Model file for the job. Use its own axes, mm. A direction names the side the tool comes from. Round coordinates to 2 decimals unless told otherwise and drop trailing zeros. Loops run counter-clockwise (first coordinate to the right, second up) from the corner with the lowest first, then second, coordinate; pieces in that order, holes last. Notation, with made-up numbers: (68, 26) - (112, 26) arc R11 ccw to (112, 31) - close; hole circle Ø7 at (65, 38). An arc over 180 degrees is marked (long way). Answer as a JSON object with one key per item and string values.
from build123d import *

# Parameters (mm, degrees)
EXTRUDE_1_DEPTH             = 25
SKETCH_2_W                  = 1
SKETCH_2_H                  = 50
CUT_EXTRUDE_1_DEPTH         = 26
SKETCH_3_W                  = 52
SKETCH_3_H                  = 1
EXTRUDE_2_DEPTH             = 25
SKETCH_4_W                  = 2
SKETCH_4_H                  = 1
EXTRUDE_3_DEPTH             = 25
SKETCH_5_W                  = 2
SKETCH_5_H                  = 1
EXTRUDE_4_DEPTH             = 25
SKETCH_6_W                  = 11
SKETCH_6_H                  = 1
CUT_EXTRUDE_2_DEPTH         = 26
SKETCH_7_R                  = 8.5
CUT_EXTRUDE_3_DEPTH         = 64
SKETCH_8_R                  = 9.5
CUT_EXTRUDE_4_DEPTH         = 5
SKETCH_9_W                  = 2
SKETCH_9_H                  = 5
EXTRUDE_5_DEPTH             = 25
HOLE_WIZARD_1_D             = 3.4
HOLE_WIZARD_1_DEPTH         = 5
HOLE_WIZARD_1_CBORE_D       = 6
HOLE_WIZARD_1_CBORE_DEPTH   = 3
SKETCH_14_R                 = 1.5
CUT_EXTRUDE_8_DEPTH         = 5
SKETCH_22_W                 = 25
SKETCH_22_H                 = 52
EXTRUDE_9_DEPTH             = 2
CUT_EXTRUDE_START           = -6
CUT_EXTRUDE_10_DEPTH        = 6
CUT_EXTRUDE_11_REACH        = 173
SKETCH_17_R                 = 7.5
CUT_EXTRUDE_12_DEPTH        = 60
HOLE_WIZARD_M3_1_D          = 2.5
HOLE_WIZARD_M3_1_DEPTH      = 8.5
HOLE_WIZARD_M3_1_TIP        = 0.751075774
HOLE_WIZARD_M3_2_AT_2_COUNT = 2
HOLE_WIZARD_M3_2_AT_2_PITCH = 8.5
HOLE_WIZARD_M3_2_AT_3_COUNT = 2
HOLE_WIZARD_M3_2_AT_3_PITCH = 17


with BuildPart() as part:
    # 草图1 → 凸台-拉伸1 (new body)
    with BuildSketch(Plane.XY):
        Polygon((-81, -29), (86, -29), (86, -34), (-86, -34), (-86, -29), (-86, 29), (-81, 29), align=None)
    extrude(amount=EXTRUDE_1_DEPTH)

    # 草图2 → 切除-拉伸1 (cut, through all)
    with BuildSketch(Plane.XY.offset(25)):
        with Locations((-85.5, 0)):
            Rectangle(SKETCH_2_W, SKETCH_2_H)
    extrude(amount=-CUT_EXTRUDE_1_DEPTH, mode=Mode.SUBTRACT)

    # 草图3 → 凸台-拉伸2 (add)
    with BuildSketch(Plane.XY.offset(25)):
        with Locations((0, -28.5)):
            Rectangle(SKETCH_3_W, SKETCH_3_H)
    extrude(amount=-EXTRUDE_2_DEPTH)

    # 草图4 → 凸台-拉伸3 (add)
    with BuildSketch(Plane.XY.offset(25)):
        with Locations((-80, -28.5)):
            Rectangle(SKETCH_4_W, SKETCH_4_H)
    extrude(amount=-EXTRUDE_3_DEPTH)

    # 草图5 → 凸台-拉伸4 (add)
    with BuildSketch(Plane.XY.offset(25)):
        with Locations((78, -28.5)):
            Rectangle(SKETCH_5_W, SKETCH_5_H)
    extrude(amount=-EXTRUDE_4_DEPTH)

    # 草图6 → 切除-拉伸2 (cut, through all)
    with BuildSketch(Plane.XY.offset(25)):
        with Locations((-20.5, -33.5)):
            Rectangle(SKETCH_6_W, SKETCH_6_H)
    cut_extrude_2 = extrude(amount=-CUT_EXTRUDE_2_DEPTH, mode=Mode.SUBTRACT)

    # 镜向1: 切除-拉伸2 across plane
    add(cut_extrude_2.mirror(Plane(origin=(0, 0, 0), x_dir=(0, 0, 1), z_dir=(1, 0, 0))), mode=Mode.SUBTRACT)

    # 草图7 → 切除-拉伸3 (cut, through all)
    with BuildSketch(Plane.XZ.offset(34)):
        with Locations((0, 12.5)):
            Circle(SKETCH_7_R)
    extrude(amount=-CUT_EXTRUDE_3_DEPTH, mode=Mode.SUBTRACT)

    # 草图8 → 切除-拉伸4 (cut)
    with BuildSketch(Plane(origin=(0, -28, 0), x_dir=(1, 0, 0), z_dir=(0, 1, 0))):
        with Locations((0, -12.5)):
            Circle(SKETCH_8_R)
    extrude(amount=-CUT_EXTRUDE_4_DEPTH, mode=Mode.SUBTRACT)

    # 草图9 → 凸台-拉伸5 (add)
    with BuildSketch(Plane(origin=(0, 0, 0), x_dir=(-1, 0, 0), z_dir=(0, 0, -1))):
        with Locations((80, 26.5)):
            Rectangle(SKETCH_9_W, SKETCH_9_H)
    extrude(amount=-EXTRUDE_5_DEPTH)

    # 孔1
    with Locations(Plane(origin=(82.5, -34, 21), x_dir=(-1, 0, 0), z_dir=(0, -1, 0))):
        with Locations((0, 0), (0, 8.5), (0, 17)):
            CounterBoreHole(HOLE_WIZARD_1_D / 2, HOLE_WIZARD_1_CBORE_D / 2, HOLE_WIZARD_1_CBORE_DEPTH, depth=HOLE_WIZARD_1_DEPTH)

    # 草图14 → 切除-拉伸8 (cut)
    with BuildSketch(Plane.XZ.offset(33)):
        with Locations((-23, 20)):
            Circle(SKETCH_14_R)
        with Locations((-23, 5)):
            Circle(SKETCH_14_R)
    cut_extrude_8 = extrude(amount=-CUT_EXTRUDE_8_DEPTH, mode=Mode.SUBTRACT)

    # 镜向2: 切除-拉伸8 across plane
    add(cut_extrude_8.mirror(Plane(origin=(0, 0, 0), x_dir=(0, 0, 1), z_dir=(1, 0, 0))), mode=Mode.SUBTRACT)

    # 草图22 → 凸台-拉伸9 (add)
    with BuildSketch(Plane(origin=(-81, 0, 0), x_dir=(0, 0, -1), z_dir=(1, 0, 0))):
        with Locations((-12.5, -2)):
            Rectangle(SKETCH_22_W, SKETCH_22_H)
    extrude(amount=EXTRUDE_9_DEPTH)

    # 草图16 → 切除-拉伸10 (cut)
    with BuildSketch(Plane.XZ.offset(34).offset(CUT_EXTRUDE_START)):
        with BuildLine():
            Line((-73, 20), (-30, 20))
            ThreePointArc((-30, 20), (-26.464466094, 18.535533906), (-25, 15))
            Line((-25, 15), (-25, 10))
            ThreePointArc((-25, 10), (-26.464466094, 6.464466094), (-30, 5))
            Line((-30, 5), (-73, 5))
            ThreePointArc((-73, 5), (-76.535533906, 6.464466094), (-78, 10))
            Line((-78, 10), (-78, 15))
            ThreePointArc((-78, 15), (-76.535533906, 18.535533906), (-73, 20))
        make_face()
    cut_extrude_10 = extrude(amount=CUT_EXTRUDE_10_DEPTH, mode=Mode.SUBTRACT)

    # 镜向3: 切除-拉伸10 across plane
    add(cut_extrude_10.mirror(Plane(origin=(0, 0, 0), x_dir=(0, 0, 1), z_dir=(1, 0, 0))), mode=Mode.SUBTRACT)

    # 草图17 → 切除-拉伸11 (cut, up to next)
    with BuildSketch(Plane.ZY.offset(85), mode=Mode.PRIVATE) as cut_extrude_11_sk1:
        with Locations((12.5, 0)):
            Circle(SKETCH_17_R)
    cut_extrude_11_tool1 = extrude(cut_extrude_11_sk1.sketch, amount=-CUT_EXTRUDE_11_REACH, mode=Mode.PRIVATE) & part.part
    add(cut_extrude_11_tool1.solids().sort_by_distance((-85, 0, 12.5))[0], mode=Mode.SUBTRACT)

    # 草图18 → 切除-拉伸12 (cut)
    with BuildSketch(Plane.XY.offset(25)):
        Polygon((-79, -29), (-86, -29), (-86, -34), (86, -34), (86, -25.759087468), (-79, -25.759087468), align=None)
    extrude(amount=-CUT_EXTRUDE_12_DEPTH, mode=Mode.SUBTRACT)

    # M3 螺纹孔1
    with Locations(Plane(origin=(-85, 21.75, 20), x_dir=(0, 0, -1), z_dir=(-1, 0, 0))):
        with Locations((0, 0), (0, 12), (10, 6), (0, 31.5), (0, 43.5), (10, 37.5)):
            Hole(HOLE_WIZARD_M3_1_D / 2, depth=HOLE_WIZARD_M3_1_DEPTH)
            with Locations((0, 0, -(HOLE_WIZARD_M3_1_DEPTH + HOLE_WIZARD_M3_1_TIP / 2))):  # 118° drill point
                Cone(0, HOLE_WIZARD_M3_1_D / 2, HOLE_WIZARD_M3_1_TIP, mode=Mode.SUBTRACT)

    # 草图24 → M3 螺纹孔2 (revolve, cut)
    with BuildSketch(Plane(origin=(-82.5, 29, 21), x_dir=(0, 0, 1), z_dir=(1, 0, 0))):
        Polygon((0, 0), (0, 5.751075774), (1.25, 5), (1.25, 0), align=None)
    hole_wizard_m3_2 = revolve(axis=Axis((-82.5, 35.35, 21), (0, -1, 0)), mode=Mode.SUBTRACT)

    # M3 螺纹孔2 at 2: M3 螺纹孔2 ×2
    with Locations(*[(0, 0, -i * HOLE_WIZARD_M3_2_AT_2_PITCH) for i in range(1, HOLE_WIZARD_M3_2_AT_2_COUNT)]):
        add(hole_wizard_m3_2, mode=Mode.SUBTRACT)

    # M3 螺纹孔2 at 3: M3 螺纹孔2 ×2
    with Locations(*[(0, 0, -i * HOLE_WIZARD_M3_2_AT_3_PITCH) for i in range(1, HOLE_WIZARD_M3_2_AT_3_COUNT)]):
        add(hole_wizard_m3_2, mode=Mode.SUBTRACT)

    # 镜向4: M3 螺纹孔2 across plane
    add(hole_wizard_m3_2.mirror(Plane.ZX), mode=Mode.SUBTRACT)

    # 镜向4 copy 1 sketch → 镜向4 copy 1 (revolve, cut)
    with BuildSketch(Plane(origin=(-82.5, -29, 12.5), x_dir=(0, 0, 1), z_dir=(1, 0, 0))):
        Polygon((0, 0), (0, -5.751075774), (1.25, -5), (1.25, 0), align=None)
    revolve(axis=Axis((-82.5, -35.35, 12.5), (0, -1, 0)), mode=Mode.SUBTRACT)

    # 镜向4 copy 2 sketch → 镜向4 copy 2 (revolve, cut)
    with BuildSketch(Plane(origin=(-82.5, -29, 4), x_dir=(0, 0, 1), z_dir=(1, 0, 0))):
        Polygon((0, 0), (0, -5.751075774), (1.25, -5), (1.25, 0), align=None)
    revolve(axis=Axis((-82.5, -35.35, 4), (0, -1, 0)), mode=Mode.SUBTRACT)


solid = part.part
1) Probe probe 1 along Z at (x, y) = (-82.5, 26.7); probe 2 along Z at (x, y) = (-80.85, 9.75); probe 3 along X at (y, z) = (26.6, 4). List the from-to ranges inside material, lowest first.
Values follow:
{"probe 1": "0 to 2.75, 5.25 to 11.25, 13.75 to 19.75, 22.25 to 25", "probe 2": "0 to 18.75, 21.25 to 25", "probe 3": "-86 to -83.75, -81.25 to -79"}
2) Slice it at B-B on y = -15.75. List the corners of the cut face in (x, z).
Values follow:
{"outline": "(-85, 0) - (-79, 0) - (-79, 8.75) - (-85, 8.75) - close; (-85, 11.25) - (-79, 11.25) - (-79, 25) - (-85, 25) - close"}
3) Tool access for faces 1 (the cylindrical face through (-83.74, 26.54, 3.84)), 2 (the flat face through (-85, -6, 7)), 3 (the cylindrical face through (-83.74, -26.54, 3.84)), 4 (the flat face through (-84, -29, 13)), 5 (the cylindrical face through (-82, 15, 9)): list every direction of +Z, -Z, +X, -X, +Y, -Y with a clear straight run to the whole face (end or side of a thin tool).
Values follow:
{"face 1": "+Y", "face 2": "+Z, -Z, -X", "face 3": "-Y", "face 4": "+Z, -Z, +X, -X, -Y", "face 5": "+X, -X"}
4) Two-plate mould, pull along Y, no slides. Class faces 6 (the cylindrical face through (-81.958, 22.229, 21.155)), 7 (the conical face through (-82.715, 23.379, 12.472)), 8 (the flat face through (-83, 0, 0)): pulls with the +Y half, pulls with the -Y half, needs draft (parallel to the pull), parting line crosses it, or undercut.
Values follow:
{"face 6": "undercut", "face 7": "pulls with the +Y half", "face 8": "needs draft"}
5) Drop flat-ended pins along their axis: P1, Ø2, axis at y = 9.75, z = 20, coming from the -X side; P2, Ø3, axis at y = -21.75, z = 20, coming from the -X side; P3, Ø2, axis at x = -82.5, z = 21, coming from the -Y side. Give the stop position or say it passes through.
Values follow:
{"P1": "through", "P2": "x = -85", "P3": "y = -23.85"}
6) Slice it at D-D on z = 7. List the corners of the cut face in (x, y), then the cut area to 3 significant figures.
Values follow:
{"outline": "(-86, -29) - (-79, -29) - (-79, -5.1) - (-85, -5.1) - (-85, -25) - (-86, -25) - close; (-86, 25) - (-85, 25) - (-85, 5.1) - (-79, 5.1) - (-79, 29) - (-86, 29) - close", "area": "295 mm²"}
7) Slice it at C-C on z = 10. List the corners of the cut face in (x, y).
Values follow:
{"outline": "(-86, -29) - (-79, -29) - (-79, -17) - (-85, -17) - (-85, -25) - (-86, -25) - close; (-86, 25) - (-85, 25) - (-85, 17) - (-79, 17) - (-79, 29) - (-86, 29) - close; (-85, -14.5) - (-79, -14.5) - (-79, -7.07) - (-85, -7.07) - close; (-85, 7.07) - (-79, 7.07) - (-79, 14.5) - (-85, 14.5) - close"}
8) Slice it at A-A on x = -80. List the corners of the cut face in (y, z).
Values follow:
{"outline": "(-29, 0) - (29, 0) - (29, 25) - (-29, 25) - close; hole circle Ø2.5 at (-21.75, 20); hole circle Ø2.5 at (-15.75, 10); hole circle Ø2.5 at (-9.75, 20); hole circle Ø15 at (0, 12.5); hole circle Ø2.5 at (9.75, 20); hole circle Ø2.5 at (15.75, 10); hole circle Ø2.5 at (21.75, 20)"}
